CAD build for the part. Positions are in the model's coordinates, mm. A direction names the side the tool comes from. Round coordinates to 2 decimals unless told otherwise and drop trailing zeros. Loops run counter-clockwise (first coordinate to the right, second up) from the corner with the lowest first, then second, coordinate; pieces in that order, holes last. Notation, with made-up numbers: (4.25, 84.5) -> (44.25, 84.5) arc R14 ccw to (44.25, 107.5) -> close; hole circle Ø2 at (-5, 81). An arc over 180 degrees is marked (long way). Answer as CSV lines item,"result".
```python
from build123d import *

# Parameters (mm, degrees)
SKETCH_R        = 8
SKETCH_R_2      = 6.5
PAD_DEPTH       = 24
CHAMFER_SIZE    = 0.5
SKETCH001_R     = 12
SKETCH001_R_2   = 6.5
PAD001_DEPTH    = 2
CHAMFER001_SIZE = 0.5
CHAMFER002_SIZE = 1
CHAMFER003_SIZE = 0.5


with BuildPart() as part:
    # Sketch → Pad (new body)
    with BuildSketch(Plane.XY):
        Circle(SKETCH_R)
        Circle(SKETCH_R_2, mode=Mode.SUBTRACT)
    extrude(amount=PAD_DEPTH)

    # Chamfer
    chamfer_edges = [part.edges().sort_by_distance(p)[0] for p in [
        (-6.5, 0, 24),
    ]]
    chamfer(chamfer_edges, length=CHAMFER_SIZE)

    # Sketch001 → Pad001 (join)
    with BuildSketch(Plane.XY):
        Circle(SKETCH001_R)
        Circle(SKETCH001_R_2, mode=Mode.SUBTRACT)
    extrude(amount=PAD001_DEPTH)

    # Chamfer001
    chamfer001_edges = [part.edges().sort_by_distance(p)[0] for p in [
        (-6.5, 0, 0),
    ]]
    chamfer(chamfer001_edges, length=CHAMFER001_SIZE)

    # Chamfer002
    chamfer002_edges = [part.edges().sort_by_distance(p)[0] for p in [
        (-12, 0, 2),
    ]]
    chamfer(chamfer002_edges, length=CHAMFER002_SIZE)

    # Chamfer003
    chamfer003_edges = [part.edges().sort_by_distance(p)[0] for p in [
        (-8, 0, 24),
    ]]
    chamfer(chamfer003_edges, length=CHAMFER003_SIZE)


solid = part.part
```
Q1. Two-plate mould, pull along X, no slides. Class faces 3 (the cylindrical face through (-5.158, -3.955, 11.839)), 4 (the cylindrical face through (-11.99, 0.53, 0.49)), 5 (the flat face through (-2, -8, 2)): pulls with the +X half, pulls with the -X half, needs draft (parallel to the pull), parting line crosses it, or undercut.
Results:
face 3,"undercut"
face 4,"parting line crosses it"
face 5,"needs draft"
Q2. Drop flat-ended pins along their axis: pin 1 Ø3 at (x, z) = (7.5, 6) entering from +Y; pin 2 Ø6 at (x, z) = (-5, 9) entering from +Y; pin 3 Ø1 at (x, z) = (3, 18.5) entering from +Y. Give the stop position or say it passes through.
Results:
pin 1,"y = 5.29"
pin 2,"y = 7.75"
pin 3,"y = 7.6"
Q3. Slice it at A-A, the plane y = 0. Give the cut face in (x, z), and give its area (4 significant figures).
Results:
outline,"(-12, 0) -> (-7, 0) -> (-6.5, 0.5) -> (-6.5, 23.5) -> (-7, 24) -> (-7.5, 24) -> (-8, 23.5) -> (-8, 2) -> (-11, 2) -> (-12, 1) -> close; (6.5, 0.5) -> (7, 0) -> (12, 0) -> (12, 1) -> (11, 2) -> (8, 2) -> (8, 23.5) -> (7.5, 24) -> (7, 24) -> (6.5, 23.5) -> close"
area,"86.25 mm2"
Q4. Tool access for faces 1 (the cylindrical face through (-1.73, -7.81, 12.6)), 2 (the flat face through (5.2, -5.2, 0)): list every direction of +Z, -Z, +X, -X, +Y, -Y with a clear straight run to the whole face (end or side of a thin tool).
Results:
face 1,"+Z"
face 2,"-Z, +X, -X, +Y, -Y"
Q5. Slice it at C-C, the plane z = 21.5. Give the cut face in (x, y), and give its area (3 significant figures).
Results:
outline,"circle Ø16 at (0, 0); hole circle Ø13 at (0, 0)"
area,"68.3 mm2"
Q6. Probe L1, parallel to Y at x = 0, z = 16.5; L2, parallel to Z at x = 8.75, y = -4; L3, parallel to X at y = -1.75, z = 9.75. List the from-to ranges inside material, lowest first. Write a range as [from, to].
Results:
L1,"[-8, -6.5], [6.5, 8]"
L2,"[0, 2]"
L3,"[-7.81, -6.26], [6.26, 7.81]"
